Verification items for this drawing (mm, ordinates from the low corner). A direction names the side the tool comes from. Give positions to 0.01 mm unless a question says otherwise; leave off trailing zeros. Loops run counter-clockwise (first coordinate to the right, second up) from the corner with the lowest first, then second, coordinate; pieces in that order, holes last. Notation, with made-up numbers: M 10.5,53 L 65.5,53 A12 ccw 65.5,58 Z; hole C 7,38 d10. An arc over 180 degrees is marked long. Use a Markdown table: item, result.
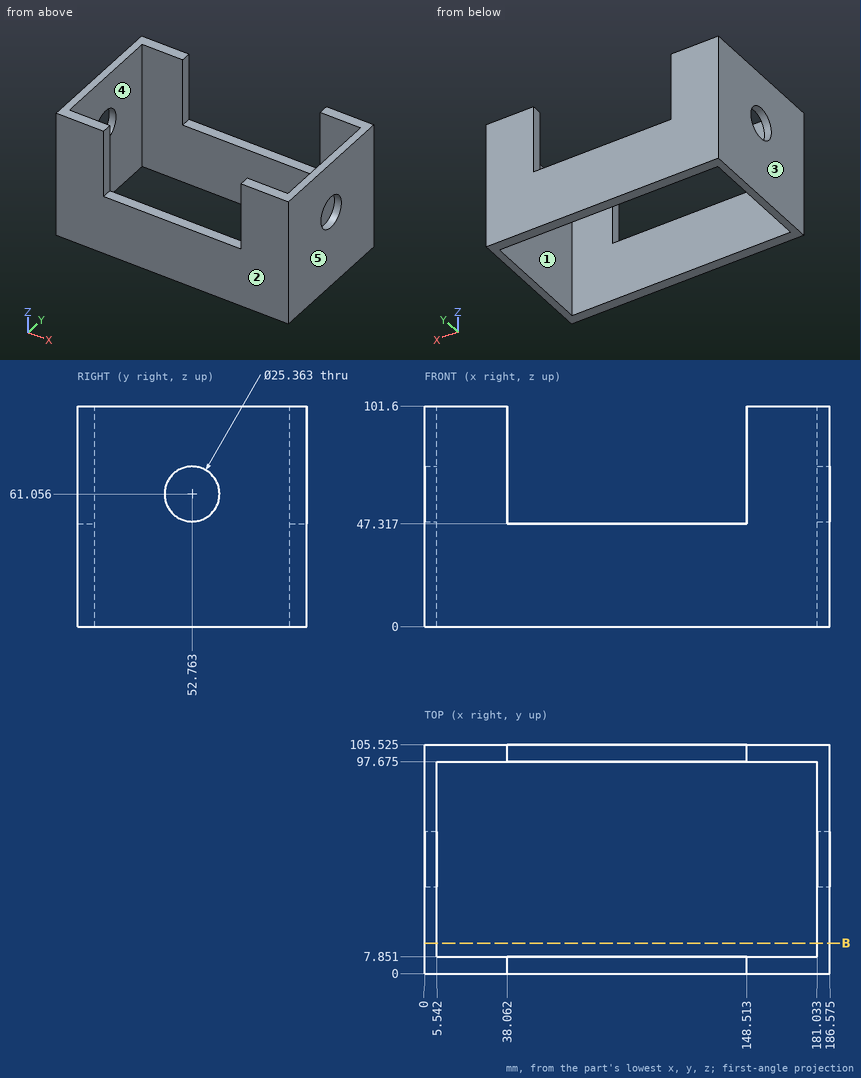
(1) Draft check along Y on the marked faces 1, 2 and 3. Enter one of: +Y half, -Y half, draft (parallel to the pull), parting line (faces both ways), or undercut.
Results below:
| item | result |
|---|---|
| face 1 | undercut |
| face 2 | -Y half |
| face 3 | draft |
(2) Set-up check for the marked faces 4 and 5: record each of +Z, -Z, +X, -X, +Y, -Y from which the full face is reachable in a straight line by a thin tool's end or side.
Results below:
| item | result |
|---|---|
| face 4 | +Z, -Z |
| face 5 | +Z, -Z, +X, +Y, -Y |
(3) Material ranges on line 1 (X direction, y = 84, z = 65) (1 decimal), recorded low to high.
Results below:
| item | result |
|---|---|
| line 1 | 0 to 5.5, 181 to 186.6 |
(4) Cross-section at B-B on y = 14. Record the cut outline in (x, z) (1 decimal).
Results below:
| item | result |
|---|---|
| outline | M 0,0 L 5.5,0 L 5.5,101.6 L 0,101.6 Z; M 181,0 L 186.6,0 L 186.6,101.6 L 181,101.6 Z |
(5) Gauge pin test, flat end, axial feed: P1, Ø2.5, axis at x = 106.5, y = 6, coming from the +Z side. Record the tip position at first contact, or that the pin passes through.
Results below:
| item | result |
|---|---|
| P1 | z = 47.32 |
